Check sheet for the drawn part. Datum: minimum x, y, z corner. Units: mm. A direction names the side the tool comes from. Give positions to 0.01 mm unless a question says otherwise; leave off trailing zeros. Loops run counter-clockwise (first coordinate to the right, second up) from the corner with the lowest first, then second, coordinate; pieces in that order, holes last. Notation, with made-up numbers: (1.25, -26.75) - (19.25, -26.75) arc R11 cw to (19.25, -12.75) - close; hole circle Ø3 at (-22, 65.25). An arc over 180 degrees is marked (long way). Answer in a Markdown table with one row per item.
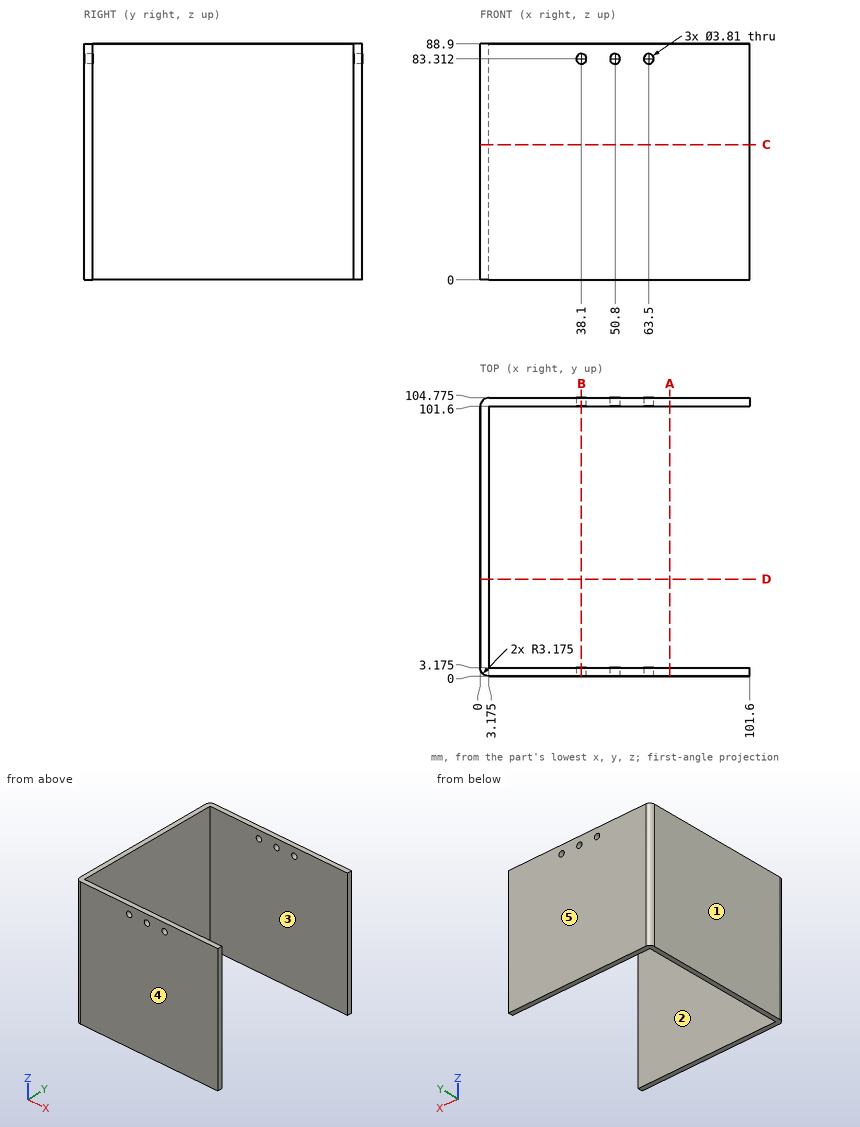
Q1. Thickness scan on line 1 (Z direction, x = 38.1, y = 103.5); line 2 (Y direction, x = 23, z = 13) (3 decimals); line 3 (X direction, y = 91, z = 41.5) (3 decimals). Record the ranges inside material, lowest first.
Completed:
| item | result |
|---|---|
| line 1 | 0 to 81.41, 85.22 to 88.9 |
| line 2 | 0 to 3.175, 101.6 to 104.775 |
| line 3 | 0 to 3.175 |
Q2. Sectioned sample at D-D (y = 36.5). Record the cut outline in (x, z) (3 decimals).
Completed:
| item | result |
|---|---|
| outline | (0, 0) - (3.175, 0) - (3.175, 88.9) - (0, 88.9) - close |
Q3. Sectioned sample at B-B (x = 38.1). Record the cut outline in (y, z) (3 decimals).
Completed:
| item | result |
|---|---|
| outline | (0, 0) - (3.175, 0) - (3.175, 81.407) - (0, 81.407) - close; (0, 85.217) - (3.175, 85.217) - (3.175, 88.9) - (0, 88.9) - close; (101.6, 0) - (104.775, 0) - (104.775, 81.407) - (101.6, 81.407) - close; (101.6, 85.217) - (104.775, 85.217) - (104.775, 88.9) - (101.6, 88.9) - close |
Q4. Tool access check on the marked faces 1 and 2. Record the directions out of +Z, -Z, +X, -X, +Y, -Y that give a thin tool (end or side, any length) a straight path to the whole face; none if there is none.
Completed:
| item | result |
|---|---|
| face 1 | +Z, -Z, -X, +Y, -Y |
| face 2 | +Z, -Z, +X |
Q5. Sectioned sample at C-C (z = 51). Record the cut outline in (x, y) (3 decimals), and give its area (3 significant figures).
Completed:
| item | result |
|---|---|
| outline | (0, 3.175) arc R3.175 ccw to (3.175, 0) - (101.6, 0) - (101.6, 3.175) - (3.175, 3.175) - (3.175, 101.6) - (101.6, 101.6) - (101.6, 104.775) - (3.175, 104.775) arc R3.175 ccw to (0, 101.6) - close |
| area | 953 mm^2 |
Q6. Draft check along Y on the marked faces 3, 4 and 5. Enter one of: +Y half, -Y half, draft (parallel to the pull), parting line (faces both ways), or undercut.
Completed:
| item | result |
|---|---|
| face 3 | undercut |
| face 4 | -Y half |
| face 5 | +Y half |
Q7. Sectioned sample at A-A (x = 71.5). Record the cut outline in (y, z) (3 decimals).
Completed:
| item | result |
|---|---|
| outline | (0, 0) - (3.175, 0) - (3.175, 88.9) - (0, 88.9) - close; (101.6, 0) - (104.775, 0) - (104.775, 88.9) - (101.6, 88.9) - close |
Q8. Go/stop test with flat-tipped pins: P1, Ø3, axis at x = 38.1, z = 83.312, coming from the -Y side; P2, Ø5, axis at y = 59.5, z = 48, coming from the +X side (3 decimals). Record where each tip stops, or that it passes through.
Completed:
| item | result |
|---|---|
| P1 | through |
| P2 | x = 3.175 |
